Input: part model. Units: mm. Frame: model coordinates. Give positions to 0.01 mm unless a question says otherwise; leave off trailing zeros. Order: outer loops, then holes, each group sorted by start corner. A loop starts at its lowest first (then second) coordinate and runs counter-clockwise, first axis right, second up.
Autodesk Inventor part; units mm, degrees
ref_plane "YZ Plane" through (0, 0, 0) normal (1, 0, 0) x (0, 1, 0)
ref_plane "XZ Plane" through (0, 0, 0) normal (0, 1, 0) x (-1, 0, 0)
ref_plane "XY Plane" through (0, 0, 0) normal (0, 0, 1) x (1, 0, 0)
sketch "Sketch1" plane through (0, 0, 0) normal (0, 1, 0) x (-1, 0, 0)
  line L0 (6.35, 3.6662) -> (6.35, -3.6662)
  line L1 (6.35, -3.6662) -> (0, -7.3323)
  line L2 (0, -7.3323) -> (-6.35, -3.6662)
  line L3 (-6.35, -3.6662) -> (-6.35, 3.6662)
  line L4 (-6.35, 3.6662) -> (0, 7.3323)
  line L5 (0, 7.3323) -> (6.35, 3.6662)
  point P0 (0, 0)
  point P1 (0, 0)
  dimension "d0" = 12.7
extrude "Extrusion1" add sketch "Sketch1" along normal blind 346.075
sketch "Sketch2" plane through (0, 0, 0) normal (0, -1, 0) x (1, 0, 0)
  circle A0 centre (0, 0) radius 2.5527
  dimension "d3" = 5.1054
extrude "Extrusion2" cut sketch "Sketch2" against normal blind 50.8
sketch "Sketch3" plane through (0, 346.075, 0) normal (0, 1, 0) x (1, 0, 0)
  circle A0 centre (0, 0) radius 2.5527
  dimension "d6" = 5.1054
extrude "Extrusion3" cut sketch "Sketch3" against normal blind 50.8
thread "Thread1"
properties part number "CORL_004_PivotShaft" material "Aluminum 6061"
1) Cut plane B-B (y = 319). Return the cut outline in (x, z), then the cut area to 3 significant figures.
2) Cut plane C-C (y = 270). Return the cut outline in (x, z).
3) Cut plane A-A (z = 0). Return the cut outline in (x, y) (3 decimals).
4) Line query: probe 1 along Z at (x, y) = (0, 14); probe 2 along X at (y, z) = (320, 0); probe 3 along Y at (x, z) = (-1.25, 2) (3 decimals). Output: solid intervals per line, ascending.
5) First-contact query: P1, Ø6, axis at x = -5, y = 244.5, coming from the +Z side; P2, Ø2, axis at y = 121.5, z = 5.5, coming from the -X side; P3, Ø4, axis at x = 0, z = 0, coming from the +Y side (3 decimals). Flat tips, straight axial feed; report the tip coordinate or a pass-through.
Geometry says:
1. outline: (-6.35, -3.67) - (0, -7.33) - (6.35, -3.67) - (6.35, 3.67) - (0, 7.33) - (-6.35, 3.67) - close; hole circle Ø5.11 at (0, 0)
1. area: 119 mm2
2. outline: (-6.35, -3.67) - (0, -7.33) - (6.35, -3.67) - (6.35, 3.67) - (0, 7.33) - (-6.35, 3.67) - close
3. outline: (-6.35, 0) - (-2.553, 0) - (-2.553, 50.8) - (2.553, 50.8) - (2.553, 0) - (6.35, 0) - (6.35, 346.075) - (2.553, 346.075) - (2.553, 295.275) - (-2.553, 295.275) - (-2.553, 346.075) - (-6.35, 346.075) - close
4. probe 1: z = -7.33 to -2.55, 2.55 to 7.33
4. probe 2: x = -6.35 to -2.55, 2.55 to 6.35
4. probe 3: y = 50.8 to 295.275
5. P1: stops at z = 6.18
5. P2: stops at x = -4.91
5. P3: stops at y = 295.275
